from build123d import *

# Parameters (mm, degrees)
SKETCH1_W          = 82.55
SKETCH1_H          = 25.4
BASE_FLANGE1_DEPTH = 0.7
EDGE_FLANGE1_DEPTH = 25.4
EDGE_FLANGE2_DEPTH = 25.4
EDGE_FLANGE3_DEPTH = 25.4
EDGE_FLANGE4_DEPTH = 25.4


# Sheet-metal steps are written as plain solids
with BuildPart() as part:
    # Sketch1 → Base-Flange1 (new body)
    with BuildSketch(Plane(origin=(0, 0, 0), x_dir=(1, 0, 0), z_dir=(0, 1, 0))):
        Rectangle(SKETCH1_W, SKETCH1_H)
    extrude(amount=-BASE_FLANGE1_DEPTH)

    # Edge-Flange1 section (across the edge) → Edge-Flange1 (add)
    with BuildSketch(Plane(origin=(42.275, -0.7, -12.7), x_dir=(-1, 0, 0), z_dir=(0, 0, 1))):
        with BuildLine():
            Line((-0.7, 1), (-0.7, 24.7))
            Line((-0.7, 24.7), (0, 24.7))
            Line((0, 24.7), (0, 1))
            ThreePointArc((0, 1), (0.292893219, 0.292893219), (1, 0))
            Line((1, 0), (1, -0.7))
            ThreePointArc((1, -0.7), (-0.202081528, -0.202081528), (-0.7, 1))
        make_face()
    extrude(amount=EDGE_FLANGE1_DEPTH)

    # Edge-Flange2 section (across the edge) → Edge-Flange2 (add)
    with BuildSketch(Plane(origin=(42.975, -26.4, 12.7), x_dir=(0, 1, 0), z_dir=(0, 0, -1))):
        with BuildLine():
            Line((-0.7, 1), (-0.7, 12))
            Line((-0.7, 12), (0, 12))
            Line((0, 12), (0, 1))
            ThreePointArc((0, 1), (0.292893219, 0.292893219), (1, 0))
            Line((1, 0), (1, -0.7))
            ThreePointArc((1, -0.7), (-0.202081528, -0.202081528), (-0.7, 1))
        make_face()
    extrude(amount=EDGE_FLANGE2_DEPTH)

    # Edge-Flange3 section (across the edge) → Edge-Flange3 (add)
    with BuildSketch(Plane(origin=(-42.275, -0.7, 12.7), x_dir=(1, 0, 0), z_dir=(0, 0, -1))):
        with BuildLine():
            Line((-0.7, 1), (-0.7, 24.7))
            Line((-0.7, 24.7), (0, 24.7))
            Line((0, 24.7), (0, 1))
            ThreePointArc((0, 1), (0.292893219, 0.292893219), (1, 0))
            Line((1, 0), (1, -0.7))
            ThreePointArc((1, -0.7), (-0.202081528, -0.202081528), (-0.7, 1))
        make_face()
    extrude(amount=EDGE_FLANGE3_DEPTH)

    # Edge-Flange4 section (across the edge) → Edge-Flange4 (add)
    with BuildSketch(Plane(origin=(-42.975, -26.4, -12.7), x_dir=(0, 1, 0), z_dir=(0, 0, 1))):
        with BuildLine():
            Line((-0.7, 1), (-0.7, 12))
            Line((-0.7, 12), (0, 12))
            Line((0, 12), (0, 1))
            ThreePointArc((0, 1), (0.292893219, 0.292893219), (1, 0))
            Line((1, 0), (1, -0.7))
            ThreePointArc((1, -0.7), (-0.202081528, -0.202081528), (-0.7, 1))
        make_face()
    extrude(amount=EDGE_FLANGE4_DEPTH)


solid = part.part
Can you work these out from the model? Positions are in its coordinate system, mm. A direction names the side the tool comes from. Coordinates: 2 decimals unless noted, no trailing zeros. Write each loop counter-clockwise with the first axis right and the second up, starting at its lowest first coordinate (ties: lowest second). Pieces come first, ordered by that corner, then holes. Notation, with made-up numbers: (16.5, 53.5) -> (51.5, 53.5) arc R21 cw to (51.5, 69.5) -> close; hole circle Ø9 at (39, 24.25). An arc over 180 degrees is marked (long way). Write item = value, one per line.
(1) Imagine slicing it at A-A (y = -9). Please give me the cut outline in (x, z) (3 decimals).
Verdict:
outline = (-42.975, -12.7) -> (-42.275, -12.7) -> (-42.275, 12.7) -> (-42.975, 12.7) -> close; (42.275, -12.7) -> (42.975, -12.7) -> (42.975, 12.7) -> (42.275, 12.7) -> close
(2) On a 3-axis mill with a long thin cutter (end or side, diameter ignored), from which of +Z, -Z, +X, -X, +Y, -Y can I reach the whole of each face in a straight line? I mean faces 1 (the face through (-49, -27.1, 0)), 2 (the face through (-1, -0.7, 0)), 3 (the face through (-42.975, -13, 0)). Say none if no direction works.
Verdict:
face_1 = +Z, -Z, +X, -X, -Y
face_2 = +Z, -Z, -Y
face_3 = +Z, -Z, -X, +Y
(3) Imagine slicing it at C-C (x = 29.5). Please give me the cut outline in (y, z), and give its area (3 significant figures).
Verdict:
outline = (-0.7, -12.7) -> (0, -12.7) -> (0, 12.7) -> (-0.7, 12.7) -> close
area = 17.8 mm^2
(4) Thinking about a two-plate mould opening in X: for faces 4 (the face through (42.275, -14, 0)), 5 (the face through (42.975, -13, 0)), 6 (the face through (50, -26.4, 0)), 7 (the face through (-42.275, -14, 0)), which applies, +X half, -X half, draft (parallel to the pull), parting line (faces both ways), or undercut?
Verdict:
face_4 = undercut
face_5 = +X half
face_6 = draft
face_7 = undercut
(5) If I drill on probe 1 along X at (y, z) = (-18, 9) (3 decimals); probe 2 along Y at (x, z) = (0, 1); probe 3 along Y at (x, z) = (-50, -11), over which ranges is the centre line in solid material (lowest first)?
Verdict:
probe_1 = -42.975 to -42.275, 42.275 to 42.975
probe_2 = -0.7 to 0
probe_3 = -27.1 to -26.4
(6) Imagine slicing it at B-B (z = -2). Please give me the cut outline in (x, y) (3 decimals).
Verdict:
outline = (-54.975, -27.1) -> (-43.975, -27.1) arc R1.7 ccw to (-42.275, -25.4) -> (-42.275, -1.7) arc R1 cw to (-41.275, -0.7) -> (41.275, -0.7) arc R1 cw to (42.275, -1.7) -> (42.275, -25.4) arc R1.7 ccw to (43.975, -27.1) -> (54.975, -27.1) -> (54.975, -26.4) -> (43.975, -26.4) arc R1 cw to (42.975, -25.4) -> (42.975, -1.7) arc R1.7 ccw to (41.275, 0) -> (-41.275, 0) arc R1.7 ccw to (-42.975, -1.7) -> (-42.975, -25.4) arc R1 cw to (-43.975, -26.4) -> (-54.975, -26.4) -> close
(7) For pin 1 (5.5 mm diameter, centred on x = -50.5, z = -5.5, fed in from +Y); pin 2 (6 mm diameter, centred on y = -21.5, z = -9.5, fed in from -X) (3 decimals); pin 3 (8 mm diameter, centred on x = 7.5, z = 2.5, fed in from -Y), each with a flat end and sliding along its axis, tell me the tip position at first contact or that it passes through.
Verdict:
pin_1 = -26.4
pin_2 = -42.975
pin_3 = -0.7
